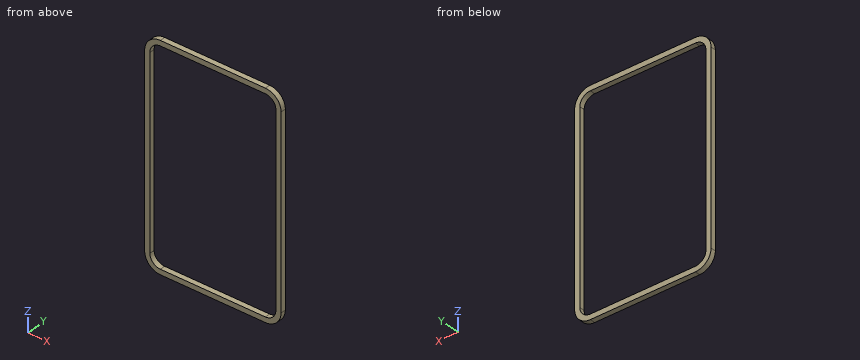
from build123d import *

# Parameters (mm, degrees)
BOX051_W     = 24
BOX051_H     = 5
BOX051_DEPTH = 40
FILLET059_R  = 2
BOX004_W     = 26
BOX004_H     = 1
BOX004_DEPTH = 42
FILLET003_R  = 3


with BuildPart() as fillet059:
    # Box051 → Box051 (new body)
    with BuildSketch(Plane(origin=(90, 4.3, 71), x_dir=(1, 0, 0), z_dir=(0, 0, 1))):
        with Locations((12, 2.5)):
            Rectangle(BOX051_W, BOX051_H)
    extrude(amount=BOX051_DEPTH)

    # Fillet059
    fillet059_edges = [fillet059.edges().sort_by_distance(p)[0] for p in [
        (90, 6.8, 111),
        (90, 6.8, 71),
        (114, 6.8, 111),
        (114, 6.8, 71),
    ]]
    fillet(fillet059_edges, radius=FILLET059_R)


with BuildPart() as fillet059_1:
    # Fillet059 placement: moved
    add(fillet059.part.moved(Location((-3, -2, 0))))


with BuildPart() as cut037:
    # Box004 → Box004 (new body)
    with BuildSketch(Plane(origin=(89, 4.3, 70), x_dir=(1, 0, 0), z_dir=(0, 0, 1))):
        with Locations((13, 0.5)):
            Rectangle(BOX004_W, BOX004_H)
    extrude(amount=BOX004_DEPTH)

    # Fillet003
    fillet003_edges = [cut037.edges().sort_by_distance(p)[0] for p in [
        (89, 4.8, 112),
        (89, 4.8, 70),
        (115, 4.8, 112),
        (115, 4.8, 70),
    ]]
    fillet(fillet003_edges, radius=FILLET003_R)


with BuildPart() as cut037_1:
    # Fillet003 placement: moved
    add(cut037.part.moved(Location((-3, -2, 0))))

    # Cut037: cut Fillet059
    add(fillet059_1.part, mode=Mode.SUBTRACT)


solid = cut037_1.part
Here's how the part is built. I have some questions about the finished solid (model axes, mm). Coordinates: 2 decimals unless noted, no trailing zeros. Write each loop counter-clockwise with the first axis right and the second up, starting at its lowest first coordinate (ties: lowest second). Pieces come first, ordered by that corner, then holes.
1) If we section it at A-A (y = 2.55): List the corners of the cut face in (x, z) for me, plus the area to 3 significant figures.
Filled in:
outline: (86, 73) arc R3 ccw to (89, 70) - (109, 70) arc R3 ccw to (112, 73) - (112, 109) arc R3 ccw to (109, 112) - (89, 112) arc R3 ccw to (86, 109) - close; hole (87, 73) arc R2 ccw to (89, 71) - (109, 71) arc R2 ccw to (111, 73) - (111, 109) arc R2 ccw to (109, 111) - (89, 111) arc R2 ccw to (87, 109) - close
area: 128 mm2
2) If I drill on line 1 (Z direction, x = 94, y = 3.1); line 2 (X direction, y = 2.65, z = 91); line 3 (Z direction, x = 88, y = 2.5), over which ranges is the centre line in solid material (lowest first)?
Filled in:
line 1: z = 70 to 71, 111 to 112
line 2: x = 86 to 87, 111 to 112
line 3: z = 70.17 to 71.27, 110.73 to 111.83
3) If we section it at B-B (x = 107): List the corners of the cut face in (y, z) for me.
Filled in:
outline: (2.3, 70) - (3.3, 70) - (3.3, 71) - (2.3, 71) - close; (2.3, 111) - (3.3, 111) - (3.3, 112) - (2.3, 112) - close
4) If we section it at C-C (z = 78): List the corners of the cut face in (x, y) for me, plus the area to 3 significant figures.
Filled in:
outline: (86, 2.3) - (87, 2.3) - (87, 3.3) - (86, 3.3) - close; (111, 2.3) - (112, 2.3) - (112, 3.3) - (111, 3.3) - close
area: 2.00 mm2
